Part print with two shaded views. Sizes in mm from the minimum x, y, z corner. Give positions to 0.01 mm unless a question says otherwise; leave off trailing zeros. Write each loop counter-clockwise with the first axis right and the second up, starting at its lowest first coordinate (ties: lowest second). Pieces come first, ordered by that corner, then holes. Notation, with made-up numbers: (-15, -35) -> (25, -35) arc R20 ccw to (25, -5) -> close; hole circle Ø1 at (38.25, -28.75). An arc over 180 degrees is marked (long way). Answer in a Markdown table with one row per item. Add a question column.
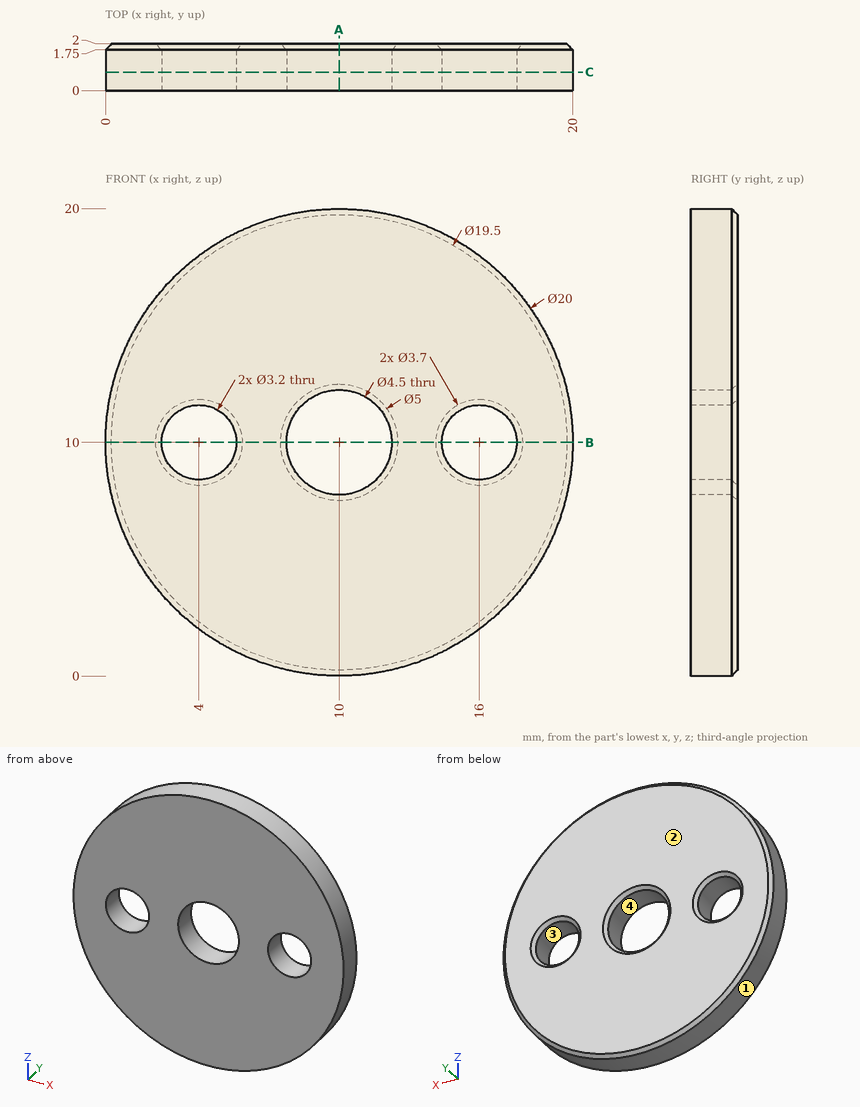
Item 1: Probe L1, parallel to X at y = 0.6, z = 10; L2, parallel to Z at x = 17.25, y = 1.8; L3, parallel to Z at x = 16.25, y = 0.45. List the from-to ranges inside material, lowest first. Write a range as from..to.
Item 2: Slice it at A-A, the plane x = 10. List the corners of the cut face in (y, z).
Item 3: Slice it at B-B, the plane z = 10. List the corners of the cut face in (x, y), then the cut area to 4 significant figures.
Item 4: Drop a flat-ended pin along its axis: pin 1 Ø2.5 at (x, z) = (16, 10) entering from -Y. Give the stop position or say it passes through.
Item 5: Slice it at C-C, the plane y = 0.8. List the corners of the cut face in (x, z).
Item 6: Mould opens along X. For the marked faces 1, 2, 3 and 4 say: released by +X, released by -X, zero draft, split by the parting line, or undercut.
Answer key:
| question | item | result |
|---|---|---|
| 1 | L1 | x = 0..2.4, 5.6..7.75, 12.25..14.4, 17.6..20 |
| 1 | L2 | z = 3.19..8.92, 11.08..16.81 |
| 1 | L3 | z = 2.19..8.42, 11.58..17.81 |
| 2 | outline | (0, 0) -> (1.75, 0) -> (2, 0.25) -> (2, 7.5) -> (1.75, 7.75) -> (0, 7.75) -> close; (0, 12.25) -> (1.75, 12.25) -> (2, 12.5) -> (2, 19.75) -> (1.75, 20) -> (0, 20) -> close |
| 3 | outline | (0, 0) -> (2.4, 0) -> (2.4, 1.75) -> (2.15, 2) -> (0.25, 2) -> (0, 1.75) -> close; (5.6, 0) -> (7.75, 0) -> (7.75, 1.75) -> (7.5, 2) -> (5.85, 2) -> (5.6, 1.75) -> close; (12.25, 0) -> (14.4, 0) -> (14.4, 1.75) -> (14.15, 2) -> (12.5, 2) -> (12.25, 1.75) -> close; (17.6, 0) -> (20, 0) -> (20, 1.75) -> (19.75, 2) -> (17.85, 2) -> (17.6, 1.75) -> close |
| 3 | area | 17.95 mm² |
| 4 | pin 1 | passes through |
| 5 | outline | circle Ø20 at (10, 10); hole circle Ø3.2 at (4, 10); hole circle Ø4.5 at (10, 10); hole circle Ø3.2 at (16, 10) |
| 6 | face 1 | split by the parting line |
| 6 | face 2 | zero draft |
| 6 | face 3 | undercut |
| 6 | face 4 | undercut |
